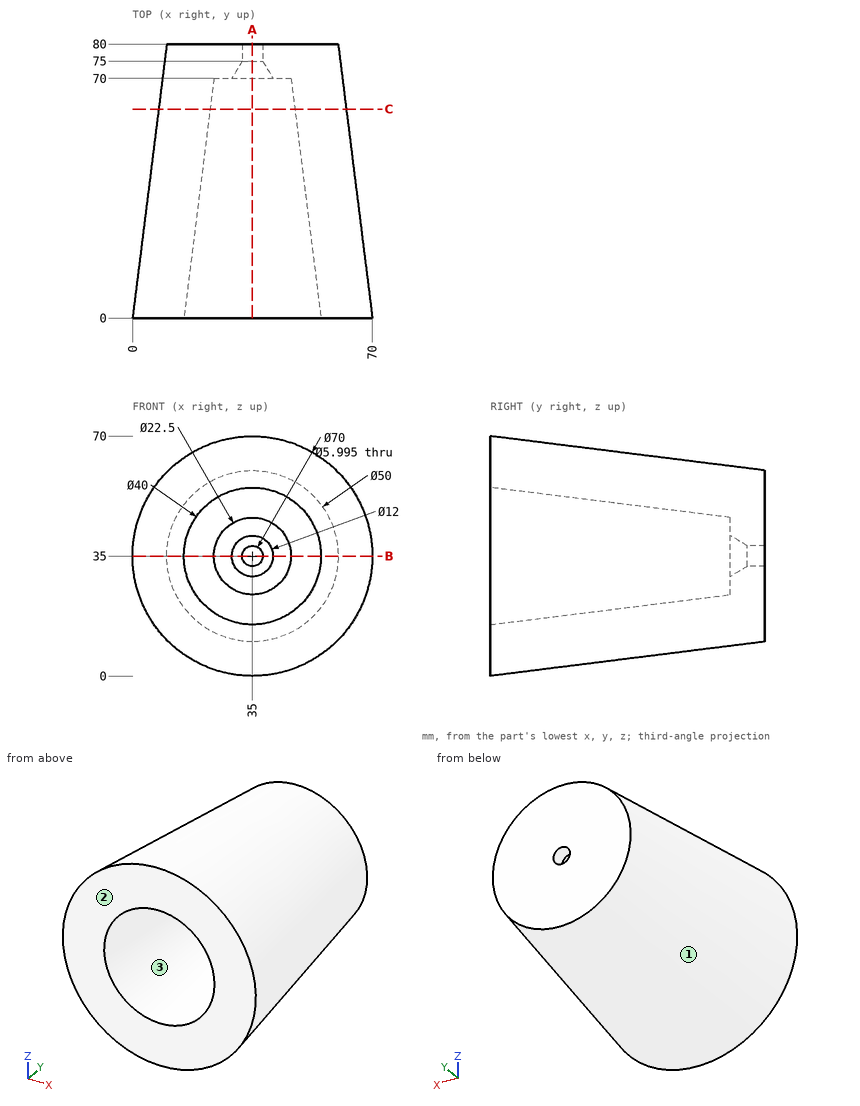
Source: three-view drawing plus pictorial views. Frame: mm from the lowest corner of the part. Round coordinates to 2 decimals unless told otherwise and drop trailing zeros. Write each loop counter-clockwise with the first axis right and the second up, starting at its lowest first coordinate (ties: lowest second). Pieces come first, ordered by that corner, then holes. Notation, with made-up numbers: M 85,46 L 120,46 A20 ccw 120,78 Z; hole C -40,-27.75 d9. An arc over 180 degrees is marked long. One line per item, written item: value. Start each with the question number.
Item 1: Mould query, pull axis Z, two halves, no side actions, for the marked faces 1, 2 and 3. Classes: pulls with the +Z half, pulls with the -Z half, needs draft (parallel to the pull), parting line crosses it, or undercut.
Item 2: Section query B-B (z = 35). Return the cut outline in (x, y).
Item 3: Pin query (flat end, axial travel): pin 1 (12 mm diameter, centred on x = 32, y = 10, fed in from +Z); pin 2 (8 mm diameter, centred on x = 48, y = 67.5, fed in from -Z); pin 3 (3 mm diameter, centred on y = 45, z = 16.5, fed in from -X). Return the tip coordinate at first contact, or that it passes through.
Item 4: Section query C-C (y = 61). Return the cut outline in (x, z) (3 decimals), plus the area to 3 significant figures.
Item 5: Section query A-A (x = 35). Return the cut outline in (y, z), plus the area to 3 significant figures.
Item 6: Ray query, L1, parallel to Z at x = 35, y = 77 (1 decimal); L2, parallel to Z at x = 35, y = 78.7. Return the intervals inside material, ascending. Write a range as from..to.
Result set:
1. face 1: parting line crosses it
1. face 2: needs draft
1. face 3: undercut
2. outline: M 0,0 L 15,0 L 23.75,70 L 29,70 L 32,75 L 32,80 L 10,80 Z; M 38,75 L 41,70 L 46.25,70 L 55,0 L 70,0 L 60,80 L 38,80 Z
3. pin 1: stops at z = 69.44
3. pin 2: stops at z = 9.91
3. pin 3: stops at x = 11.02
4. outline: C 35,35 d54.75; hole C 35,35 d24.75
4. area: 1,870 mm²
5. outline: M 0,0 L 80,10 L 80,32 L 75,32 L 70,29 L 70,23.75 L 0,15 Z; M 0,55 L 70,46.25 L 70,41 L 75,38 L 80,38 L 80,60 L 0,70 Z
5. area: 2,540 mm²
6. L1: z = 9.6..32, 38..60.4
6. L2: z = 9.84..32, 38..60.16
